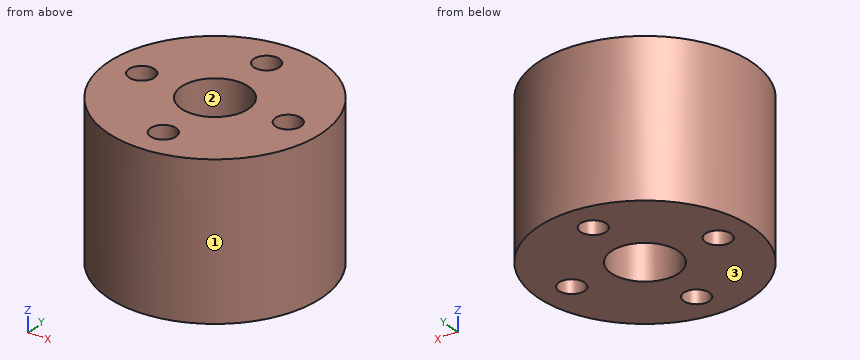
```python
from build123d import *

# Parameters (mm, degrees)
SKETCH1_R           = 60
SKETCH1_R_2         = 5.5
SKETCH1_R_3         = 9
BOSS_EXTRUDE1_DEPTH = 25
CUT_EXTRUDE7_REACH  = 90.459
SKETCH6_R           = 2.1
CIRPATTERN4_COUNT   = 4
SKETCH2_R           = 63
SKETCH2_R_2         = 60
BOSS_EXTRUDE2_DEPTH = 300
SKETCH3_R           = 11.04
CUT_EXTRUDE1_DEPTH  = 10
CUT_EXTRUDE2_REACH  = 314.95
SKETCH4_R           = 1.5
CIRPATTERN1_COUNT   = 4
CUT_EXTRUDE3_DEPTH  = 3
CIRPATTERN2_COUNT   = 4
SKETCH7_OUTSIDE_W   = 197.786
SKETCH7_OUTSIDE_H   = 197.786
SKETCH7_OUTSIDE_R   = 17.5
CUT_EXTRUDE8_DEPTH  = 313.950475315


with BuildPart() as part:
    # Sketch1 → Boss-Extrude1 (new body)
    with BuildSketch(Plane.XY):
        Circle(SKETCH1_R)
        with Locations((25, 0)):
            Circle(SKETCH1_R_2, mode=Mode.SUBTRACT)
        with Locations((-25, 0)):
            Circle(SKETCH1_R_3, mode=Mode.SUBTRACT)
    extrude(amount=-BOSS_EXTRUDE1_DEPTH)

    # Sketch6 → Cut-Extrude7 (cut, up to next)
    with BuildSketch(Plane.XY, mode=Mode.PRIVATE) as cut_extrude7_sk1:
        with Locations((25, 12)):
            Circle(SKETCH6_R)
    cut_extrude7_tool1 = extrude(cut_extrude7_sk1.sketch, amount=-CUT_EXTRUDE7_REACH, mode=Mode.PRIVATE) & part.part
    cut_extrude7 = cut_extrude7_tool1.solids().sort_by_distance((25, 12, 0))[0]
    add(cut_extrude7, mode=Mode.SUBTRACT)

    # CirPattern4: Cut-Extrude7 ×4 about axis
    cirpattern4_axis = Axis((25, 0, 0), (0, 0, 1))
    for i in range(1, CIRPATTERN4_COUNT):
        add(cut_extrude7.rotate(cirpattern4_axis, i * 360 / CIRPATTERN4_COUNT), mode=Mode.SUBTRACT)

    # Sketch2 → Boss-Extrude2 (add)
    with BuildSketch(Plane.XY):
        Circle(SKETCH2_R)
        Circle(SKETCH2_R_2, mode=Mode.SUBTRACT)
    extrude(amount=-BOSS_EXTRUDE2_DEPTH)

    # Sketch3 → Cut-Extrude1 (cut)
    with BuildSketch(Plane(origin=(0, 0, -25), x_dir=(-1, 0, 0), z_dir=(0, 0, -1))):
        with Locations((25, 0)):
            Circle(SKETCH3_R)
    extrude(amount=-CUT_EXTRUDE1_DEPTH, mode=Mode.SUBTRACT)

    # Sketch4 → Cut-Extrude2 (cut, up to next)
    with BuildSketch(Plane.XY, mode=Mode.PRIVATE) as cut_extrude2_sk1:
        with Locations((-39, 0)):
            Circle(SKETCH4_R)
    cut_extrude2_tool1 = extrude(cut_extrude2_sk1.sketch, amount=-CUT_EXTRUDE2_REACH, mode=Mode.PRIVATE) & part.part
    cut_extrude2 = cut_extrude2_tool1.solids().sort_by_distance((-39, 0, 0))[0]
    add(cut_extrude2, mode=Mode.SUBTRACT)

    # CirPattern1: Cut-Extrude2 ×4 about axis
    cirpattern1_axis = Axis((-25, 0, 0), (0, 0, 1))
    for i in range(1, CIRPATTERN1_COUNT):
        add(cut_extrude2.rotate(cirpattern1_axis, i * 360 / CIRPATTERN1_COUNT), mode=Mode.SUBTRACT)

    # Sketch5 → Cut-Extrude3 (cut)
    with BuildSketch(Plane.XY):
        Polygon((-12.732050808, -3), (-9.267949192, -3), (-7.535898385, 0), (-9.267949192, 3), (-12.732050808, 3), (-14.464101615, 0), align=None)
    cut_extrude3 = extrude(amount=-CUT_EXTRUDE3_DEPTH, mode=Mode.SUBTRACT)

    # CirPattern2: Cut-Extrude3 ×4 about axis
    cirpattern2_axis = Axis((-25, 0, 0), (0, 0, 1))
    for i in range(1, CIRPATTERN2_COUNT):
        add(cut_extrude3.rotate(cirpattern2_axis, i * 360 / CIRPATTERN2_COUNT), mode=Mode.SUBTRACT)

    # Sketch7 outside → Cut-Extrude8 (cut, through all)
    with BuildSketch(Plane.XY):
        Rectangle(SKETCH7_OUTSIDE_W, SKETCH7_OUTSIDE_H)
        with Locations((25, 0)):
            Circle(SKETCH7_OUTSIDE_R, mode=Mode.SUBTRACT)
    extrude(amount=-CUT_EXTRUDE8_DEPTH, mode=Mode.SUBTRACT)


solid = part.part
```
Input: part model. Units: mm. Frame: model coordinates. Face numbers are marked on the shaded views. Give positions to 0.01 mm unless a question says otherwise; leave off trailing zeros. Order: outer loops, then holes, each group sorted by start corner. A loop starts at its lowest first (then second) coordinate and runs counter-clockwise, first axis right, second up. Notation, with made-up numbers: M -17.75,52.25 L 10.25,52.25 A12 ccw 10.25,74.25 Z; hole C -20,67 d3. An arc over 180 degrees is marked long. One line per question, with ' | ' between items.
1) Draft query along Y for the marked faces 1, 2 and 3. Return one class per face: pulls with the +Y half, pulls with the -Y half, needs draft (parallel to the pull), parting line crosses it, or undercut.
Filled in:
face 1: parting line crosses it | face 2: undercut | face 3: needs draft
2) Section C-C on x = 37. Output: boundary loops of the cut face in (y, z).
Filled in:
outline: M -12.74,-25 L -2.1,-25 L -2.1,0 L -12.74,0 Z; M 2.1,-25 L 12.74,-25 L 12.74,0 L 2.1,0 Z
3) Section D-D on y = 12. Output: boundary loops of the cut face in (x, z), and give its area (3 significant figures).
Filled in:
outline: M 12.26,-25 L 22.9,-25 L 22.9,0 L 12.26,0 Z; M 27.1,-25 L 37.74,-25 L 37.74,0 L 27.1,0 Z | area: 532 mm2
4) Contact query for flat-ended pins moving along their axis: P1, Ø5.5, axis at x = 13, y = 0, coming from the -Z side; P2, Ø1, axis at y = -11.5, z = -14, coming from the +X side; P3, Ø1.5, axis at x = 33.5, z = -15.5, coming from the -Y side; P4, Ø2, axis at x = 20.5, z = -14.5, coming from the -Y side. Output: stop coordinate, or through.
Filled in:
P1: stops at z = -25 | P2: stops at x = 38.61 | P3: stops at y = -15.69 | P4: stops at y = -17.15
5) Ray query, L1, parallel to Y at x = 25, z = -16.5; L2, parallel to Y at x = 20, z = -4.5; L3, parallel to Y at x = 22, z = -4. Return the intervals inside material, ascending.
Filled in:
L1: y = -17.5 to -14.1, -9.9 to -5.5, 5.5 to 9.9, 14.1 to 17.5 | L2: y = -16.77 to -2.29, 2.29 to 16.77 | L3: y = -17.24 to -4.61, 4.61 to 17.24
6) Section B-B on z = -21.75. Output: boundary loops of the cut face in (x, y), and give its area (3 significant figures).
Filled in:
outline: C 25,0 d35; hole C 13,0 d4.2; hole C 25,0 d11; hole C 25,-12 d4.2; hole C 25,12 d4.2; hole C 37,0 d4.2 | area: 812 mm2
7) Section A-A on y = 0. Output: boundary loops of the cut face in (x, z), and give its area (3 significant figures).
Filled in:
outline: M 7.5,-25 L 10.9,-25 L 10.9,0 L 7.5,0 Z; M 15.1,-25 L 19.5,-25 L 19.5,0 L 15.1,0 Z; M 30.5,-25 L 34.9,-25 L 34.9,0 L 30.5,0 Z; M 39.1,-25 L 42.5,-25 L 42.5,0 L 39.1,0 Z | area: 390 mm2
